Model file for the job. Use its own axes, mm. Face numbers are marked on the shaded views. A direction names the side the tool comes from. Give positions to 0.01 mm unless a question says otherwise; leave off trailing zeros. Write each loop counter-clockwise with the first axis right and the second up, starting at its lowest first coordinate (ties: lowest second). Pieces come first, ordered by that corner, then holes. Notation, with made-up numbers: (68, -3.75) - (72, -3.75) arc R12 cw to (72, 17.25) - close; hole circle Ø5 at (-7.75, -4.75). An arc over 180 degrees is marked (long way). One line per item, written item: value. Start each with the question number.
(1) Mould opens along X. For the marked faces 3 and 4 say: pulls with the +X half, pulls with the -X half, needs draft (parallel to the pull), parting line crosses it, or undercut.
(2) Cut at C-C, the plane z = 7.5. List the corners of the cut face in (x, y), and give its area (3 significant figures).
(3) Probe L1, parallel to X at y = 0.5, z = 34; L2, parallel to Z at x = 28.5, y = -6.25 (3 decimals); L3, parallel to X at y = 4.25, z = 7. List the from-to ranges inside material, lowest first.
(4) Cut at A-A, the plane y = 0. List the corners of the cut face in (x, z) (3 decimals).
(5) 3-axis set-ups, long thin cutter, end or side, ignore diameter. For the marked faces 1 and 2: which of +Z, -Z, +X, -X, +Y, -Y reach the whole face in a straight line?
(6) Cut at D-D, the plane y = -4. List the corners of the cut face in (x, z) (3 decimals), and give its area (3 significant figures).
(7) Drop flat-ended pins along their axis: P1, Ø6, axis at y = -6.5, z = 55, coming from the -X side; P2, Ø2, axis at y = -5, z = 8.5, coming from the +X side; P3, Ø1.5, axis at x = 36.5, z = 8, coming from the +Y side. Give the stop position or say it passes through.
(8) Cut at B-B, the plane x = 38.1. List the corners of the cut face in (y, z) (3 decimals), and give its area (3 significant figures).
from build123d import *

# Parameters (mm, degrees)
SKETCH1_R           = 9
BOSS_EXTRUDE1_DEPTH = 65
LPATTERN1_COUNT     = 3
LPATTERN1_PITCH     = 19.05
SKETCH2_W           = 63.5
SKETCH2_H           = 19.05
BOSS_EXTRUDE5_DEPTH = 3.175
LPATTERN2_COUNT     = 2
LPATTERN2_PITCH     = 68.175


with BuildPart() as part:
    # Sketch1 → Boss-Extrude1 (new body)
    with BuildSketch(Plane.XY):
        Circle(SKETCH1_R)
    extrude(amount=BOSS_EXTRUDE1_DEPTH)


with BuildPart() as lpattern1_1:
    # LPattern1: pattern copy
    add(part.part.moved(Location(Vector(1, 0, 0) * (1 * LPATTERN1_PITCH))))


with BuildPart() as lpattern1_2:
    # LPattern1: pattern copy
    add(part.part.moved(Location(Vector(1, 0, 0) * (2 * LPATTERN1_PITCH))))


with BuildPart() as part_1:
    add(part.part)

    add(lpattern1_1.part)  # Boss-Extrude5 merges LPattern1_1

    add(lpattern1_2.part)  # Boss-Extrude5 merges LPattern1_2
    # Sketch2 → Boss-Extrude5 (add)
    with BuildSketch(Plane(origin=(0, 0, 0), x_dir=(-1, 0, 0), z_dir=(0, 0, -1))):
        with Locations((-19.05, 0)):
            Rectangle(SKETCH2_W, SKETCH2_H)
    boss_extrude5 = extrude(amount=BOSS_EXTRUDE5_DEPTH)

    # LPattern2: Boss-Extrude5 ×2
    with Locations(*[(0, 0, i * LPATTERN2_PITCH) for i in range(1, LPATTERN2_COUNT)]):
        add(boss_extrude5)


solid = part_1.part
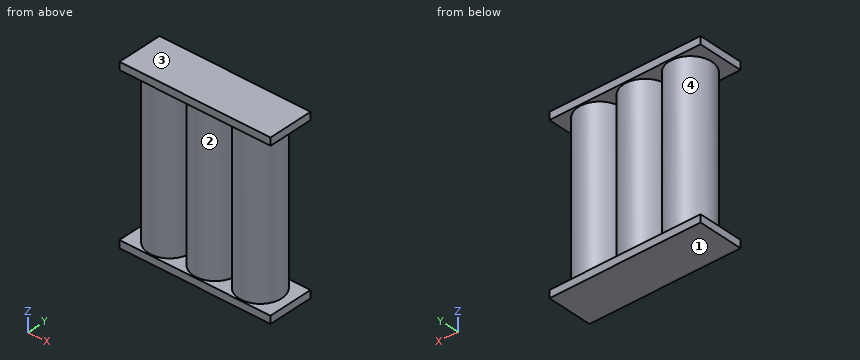
Answers follow:
1. face 3: needs draft
1. face 4: undercut
2. outline: circle Ø18 at (0, 0); circle Ø18 at (19.05, 0); circle Ø18 at (38.1, 0)
2. area: 763 mm²
3. L1: x = -8.99 to 8.99, 10.06 to 28.04, 29.11 to 47.09
3. L2: z = -3.175 to 0, 65 to 68.175
3. L3: x = -7.93 to 7.93, 11.12 to 26.98, 30.17 to 46.03
4. outline: (-12.7, -3.175) - (50.8, -3.175) - (50.8, 0) - (47.1, 0) - (47.1, 65) - (50.8, 65) - (50.8, 68.175) - (-12.7, 68.175) - (-12.7, 65) - (-9, 65) - (-9, 0) - (-12.7, 0) - close; hole (9, 0) - (10.05, 0) - (10.05, 65) - (9, 65) - close; hole (28.05, 0) - (29.1, 0) - (29.1, 65) - (28.05, 65) - close
5. face 1: -Z, +X, -X, +Y, -Y
5. face 2: none
6. outline: (-12.7, -3.175) - (50.8, -3.175) - (50.8, 0) - (46.162, 0) - (46.162, 65) - (50.8, 65) - (50.8, 68.175) - (-12.7, 68.175) - (-12.7, 65) - (-8.062, 65) - (-8.062, 0) - (-12.7, 0) - close; hole (8.062, 0) - (10.988, 0) - (10.988, 65) - (8.062, 65) - close; hole (27.112, 0) - (30.038, 0) - (30.038, 65) - (27.112, 65) - close
6. area: 3,550 mm²
7. P1: stops at x = -8.29
7. P2: stops at x = 46.16
7. P3: stops at y = 8.96
8. outline: (-9.525, -3.175) - (9.525, -3.175) - (9.525, 0) - (9, 0) - (9, 65) - (9.525, 65) - (9.525, 68.175) - (-9.525, 68.175) - (-9.525, 65) - (-9, 65) - (-9, 0) - (-9.525, 0) - close
8. area: 1,290 mm²
